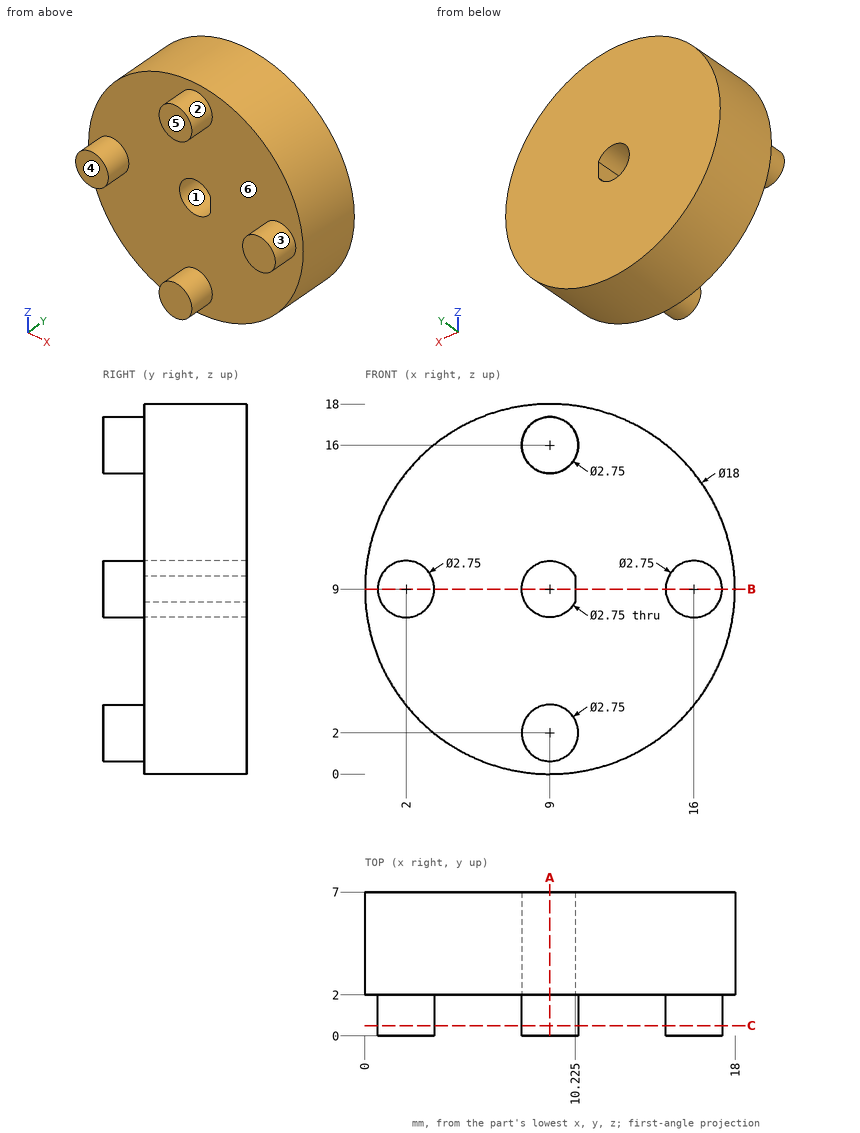
Input: dimensioned drawing with shaded views. Units: mm. Origin: part minimum x, y, z. A direction names the side the tool comes from. Give positions to 0.01 mm unless a question says otherwise; leave off trailing zeros. Order: outer loops, then holes, each group sorted by start corner. A loop starts at its lowest first (then second) coordinate and runs counter-clockwise, first axis right, second up. Notation, with made-up numbers: (24, -16) -> (41, -16) arc R10 cw to (41, -8) -> close; hole circle Ø10 at (-11, 10.5). An arc over 180 degrees is marked (long way). Answer as a JSON object with one key per item and string values.
Q1. Draft query along Z for the marked faces 1, 2, 3 and 4. Return one class per face: released by +Z, released by -Z, zero draft, split by the parting line, or undercut.
Entries:
{"face 1": "undercut", "face 2": "undercut", "face 3": "split by the parting line", "face 4": "zero draft"}
Q2. Section C-C (y = 0.5). State how many separate pieces and enclosed holes the cut face has.
Entries:
{"separate pieces": "4", "enclosed holes": "0"}
Q3. First-contact query: pin 1 (4 mm diameter, centred on x = 12, z = 15, fed in from -Y); pin 2 (1.5 mm diameter, centred on x = 14, z = 12.5, fed in from -Y). Flat tips, straight axial feed; report the tip coordinate or a pass-through.
Entries:
{"pin 1": "stops at y = 0", "pin 2": "stops at y = 2"}
Q4. Access query for the marked faces 5 and 6. Directions: +Z, -Z, +X, -X, +Y, -Y. A direction counts if a zero-diameter tool reaches every point of the face in a straight line with its end or side. Return the directions, or none.
Entries:
{"face 5": "+Z, -Z, +X, -X, -Y", "face 6": "-Y"}
Q5. Material intervals for probe 1 along Z at (x, y) = (9, 3.4) (1 decimal); probe 2 along Y at (x, z) = (7.75, 17); probe 3 along X at (y, z) = (5.25, 8.25), sorted ascending.
Entries:
{"probe 1": "z = 0 to 7.6, 10.4 to 18", "probe 2": "y = 2 to 7", "probe 3": "x = 0.03 to 7.85, 10.15 to 17.97"}
Q6. Section B-B (z = 9). Output: boundary loops of the cut face in (x, y) (1 decimal), plus the area to 3 significant figures.
Entries:
{"outline": "(0, 2) -> (0.6, 2) -> (0.6, 0) -> (3.4, 0) -> (3.4, 2) -> (7.6, 2) -> (7.6, 7) -> (0, 7) -> close; (10.2, 2) -> (14.6, 2) -> (14.6, 0) -> (17.4, 0) -> (17.4, 2) -> (18, 2) -> (18, 7) -> (10.2, 7) -> close", "area": "88.0 mm^2"}
Q7. Section A-A (x = 9). Output: boundary loops of the cut face in (y, z) (1 decimal).
Entries:
{"outline": "(0, 0.6) -> (2, 0.6) -> (2, 0) -> (7, 0) -> (7, 7.6) -> (2, 7.6) -> (2, 3.4) -> (0, 3.4) -> close; (0, 14.6) -> (2, 14.6) -> (2, 10.4) -> (7, 10.4) -> (7, 18) -> (2, 18) -> (2, 17.4) -> (0, 17.4) -> close"}
